Part model, mm, in its own coordinate system. A direction names the side the tool comes from. Coordinates: 2 decimals unless noted, no trailing zeros. Order: outer loops, then holes, each group sorted by start corner. A loop starts at its lowest first (then second) coordinate and runs counter-clockwise, first axis right, second up.
from build123d import *

# Parameters (mm, degrees)
SPUR_START             = -34.654843931
SPUR_GEAR_AM_OUTLINE_R = 5
SPUR_GEAR_AM_DEPTH     = 6
BOSS_EXTRUDE1_START    = -6
SKETCH2_R              = 5
SKETCH2_R_2            = 3
BOSS_EXTRUDE1_DEPTH    = 6
CUT_EXTRUDE1_REACH     = 65.242
SKETCH3_R              = 3.4


# Read off the part's stored shape, not the designer's step: spur gear_am
with BuildPart() as part:
    # spur gear_am outline → spur gear_am (new body)
    with BuildSketch(Plane.YZ.offset(SPUR_START)):
        with BuildLine():
            ThreePointArc((-3.907949552, 51.357822977), (-4.560317936, 51.46921073), (-5.215177847, 51.564867598))
            ThreePointArc((-5.215177847, 51.564867598), (-6.830693003, 49.038493172), (-7.624540457, 46.146735372))
            ThreePointArc((-7.624540457, 46.146735372), (-8.862265725, 46.181781364), (-10.099990992, 46.146735372))
            ThreePointArc((-10.099990992, 46.146735372), (-10.893838446, 49.038493172), (-12.509353602, 51.564867598))
            ThreePointArc((-12.509353602, 51.564867598), (-13.164213513, 51.46921073), (-13.816581897, 51.357822977))
            ThreePointArc((-13.816581897, 51.357822977), (-14.572335481, 48.455876478), (-14.433726972, 45.460339024))
            ThreePointArc((-14.433726972, 45.460339024), (-15.62170346, 45.111191601), (-16.788020333, 44.69538274))
            ThreePointArc((-16.788020333, 44.69538274), (-18.436616432, 47.200295486), (-20.75375528, 49.103798708))
            ThreePointArc((-20.75375528, 49.103798708), (-21.347004468, 48.810460779), (-21.933022961, 48.502931813))
            ThreePointArc((-21.933022961, 48.502931813), (-21.755036547, 45.509475985), (-20.69754004, 42.703382954))
            ThreePointArc((-20.69754004, 42.703382954), (-21.719480333, 42.004219099), (-22.700221591, 41.248349637))
            ThreePointArc((-22.700221591, 41.248349637), (-25.042190262, 43.121219015), (-27.834135107, 44.215522876))
            ThreePointArc((-27.834135107, 44.215522876), (-28.307702207, 43.753217846), (-28.770007237, 43.279650746))
            ThreePointArc((-28.770007237, 43.279650746), (-27.675703376, 40.487705901), (-25.802833998, 38.145737231))
            ThreePointArc((-25.802833998, 38.145737231), (-26.558703459, 37.164995972), (-27.257867315, 36.143055679))
            ThreePointArc((-27.257867315, 36.143055679), (-30.063960346, 37.200552186), (-33.057416174, 37.3785386))
            ThreePointArc((-33.057416174, 37.3785386), (-33.36494514, 36.792520107), (-33.658283069, 36.199270919))
            ThreePointArc((-33.658283069, 36.199270919), (-31.754779846, 33.882132071), (-29.249867101, 32.233535972))
            ThreePointArc((-29.249867101, 32.233535972), (-29.665675962, 31.067219099), (-30.014823385, 29.879242611))
            ThreePointArc((-30.014823385, 29.879242611), (-33.010360839, 30.01785112), (-35.912307338, 29.262097536))
            ThreePointArc((-35.912307338, 29.262097536), (-36.023695091, 28.609729152), (-36.119351959, 27.954869241))
            ThreePointArc((-36.119351959, 27.954869241), (-33.592977533, 26.339354085), (-30.701219732, 25.545506631))
            ThreePointArc((-30.701219732, 25.545506631), (-30.736265724, 24.307781363), (-30.701219732, 23.070056096))
            ThreePointArc((-30.701219732, 23.070056096), (-33.592977533, 22.276208642), (-36.119351959, 20.660693486))
            ThreePointArc((-36.119351959, 20.660693486), (-36.023695091, 20.005833575), (-35.912307338, 19.353465191))
            ThreePointArc((-35.912307338, 19.353465191), (-33.010360839, 18.597711607), (-30.014823385, 18.736320117))
            ThreePointArc((-30.014823385, 18.736320117), (-29.665675962, 17.548343629), (-29.249867101, 16.382026755))
            ThreePointArc((-29.249867101, 16.382026755), (-31.754779846, 14.733430656), (-33.658283069, 12.416291808))
            ThreePointArc((-33.658283069, 12.416291808), (-33.36494514, 11.82304262), (-33.057416174, 11.237024127))
            ThreePointArc((-33.057416174, 11.237024127), (-30.063960346, 11.415010541), (-27.257867315, 12.472507048))
            ThreePointArc((-27.257867315, 12.472507048), (-26.558703459, 11.450566755), (-25.802833998, 10.469825497))
            ThreePointArc((-25.802833998, 10.469825497), (-27.675703376, 8.127856826), (-28.770007237, 5.335911981))
            ThreePointArc((-28.770007237, 5.335911981), (-28.307702207, 4.862344881), (-27.834135107, 4.400039851))
            ThreePointArc((-27.834135107, 4.400039851), (-25.042190262, 5.494343712), (-22.700221591, 7.36721309))
            ThreePointArc((-22.700221591, 7.36721309), (-21.719480333, 6.611343629), (-20.69754004, 5.912179773))
            ThreePointArc((-20.69754004, 5.912179773), (-21.755036547, 3.106086742), (-21.933022961, 0.112630914))
            ThreePointArc((-21.933022961, 0.112630914), (-21.347004468, -0.194898052), (-20.75375528, -0.488235981))
            ThreePointArc((-20.75375528, -0.488235981), (-18.436616432, 1.415267242), (-16.788020333, 3.920179987))
            ThreePointArc((-16.788020333, 3.920179987), (-15.62170346, 3.504371126), (-14.433726972, 3.155223703))
            ThreePointArc((-14.433726972, 3.155223703), (-14.572335481, 0.159686249), (-13.816581897, -2.742260249))
            ThreePointArc((-13.816581897, -2.742260249), (-13.164213513, -2.853648003), (-12.509353602, -2.949304871))
            ThreePointArc((-12.509353602, -2.949304871), (-10.893838446, -0.422930445), (-10.099990992, 2.468827356))
            ThreePointArc((-10.099990992, 2.468827356), (-8.862265725, 2.433781364), (-7.624540457, 2.468827356))
            ThreePointArc((-7.624540457, 2.468827356), (-6.830693003, -0.422930445), (-5.215177847, -2.949304871))
            ThreePointArc((-5.215177847, -2.949304871), (-4.560317936, -2.853648003), (-3.907949552, -2.742260249))
            ThreePointArc((-3.907949552, -2.742260249), (-3.152195968, 0.159686249), (-3.290804477, 3.155223703))
            ThreePointArc((-3.290804477, 3.155223703), (-2.102827989, 3.504371126), (-0.936511116, 3.920179987))
            ThreePointArc((-0.936511116, 3.920179987), (0.712084983, 1.415267242), (3.029223831, -0.488235981))
            ThreePointArc((3.029223831, -0.488235981), (3.622473019, -0.194898052), (4.208491512, 0.112630914))
            ThreePointArc((4.208491512, 0.112630914), (4.030505098, 3.106086742), (2.973008591, 5.912179773))
            ThreePointArc((2.973008591, 5.912179773), (3.994948884, 6.611343629), (4.975690142, 7.36721309))
            ThreePointArc((4.975690142, 7.36721309), (7.317658813, 5.494343712), (10.109603658, 4.400039851))
            ThreePointArc((10.109603658, 4.400039851), (10.583170758, 4.862344881), (11.045475788, 5.335911981))
            ThreePointArc((11.045475788, 5.335911981), (9.951171927, 8.127856826), (8.078302549, 10.469825497))
            ThreePointArc((8.078302549, 10.469825497), (8.83417201, 11.450566755), (9.533335866, 12.472507048))
            ThreePointArc((9.533335866, 12.472507048), (12.339428897, 11.415010541), (15.332884725, 11.237024127))
            ThreePointArc((15.332884725, 11.237024127), (15.640413691, 11.82304262), (15.93375162, 12.416291808))
            ThreePointArc((15.93375162, 12.416291808), (14.030248397, 14.733430656), (11.525335652, 16.382026755))
            ThreePointArc((11.525335652, 16.382026755), (11.941144513, 17.548343629), (12.290291936, 18.736320117))
            ThreePointArc((12.290291936, 18.736320117), (15.28582939, 18.597711607), (18.187775889, 19.353465191))
            ThreePointArc((18.187775889, 19.353465191), (18.299163642, 20.005833575), (18.39482051, 20.660693486))
            ThreePointArc((18.39482051, 20.660693486), (15.868446084, 22.276208642), (12.976688283, 23.070056096))
            ThreePointArc((12.976688283, 23.070056096), (13.011734276, 24.307781363), (12.976688283, 25.545506631))
            ThreePointArc((12.976688283, 25.545506631), (15.868446084, 26.339354085), (18.39482051, 27.954869241))
            ThreePointArc((18.39482051, 27.954869241), (18.299163642, 28.609729152), (18.187775889, 29.262097536))
            ThreePointArc((18.187775889, 29.262097536), (15.28582939, 30.01785112), (12.290291936, 29.879242611))
            ThreePointArc((12.290291936, 29.879242611), (11.941144513, 31.067219099), (11.525335652, 32.233535972))
            ThreePointArc((11.525335652, 32.233535972), (14.030248397, 33.882132071), (15.93375162, 36.199270919))
            ThreePointArc((15.93375162, 36.199270919), (15.640413691, 36.792520107), (15.332884725, 37.3785386))
            ThreePointArc((15.332884725, 37.3785386), (12.339428897, 37.200552186), (9.533335866, 36.143055679))
            ThreePointArc((9.533335866, 36.143055679), (8.83417201, 37.164995972), (8.078302549, 38.145737231))
            ThreePointArc((8.078302549, 38.145737231), (9.951171927, 40.487705901), (11.045475788, 43.279650746))
            ThreePointArc((11.045475788, 43.279650746), (10.583170758, 43.753217846), (10.109603658, 44.215522876))
            ThreePointArc((10.109603658, 44.215522876), (7.317658813, 43.121219015), (4.975690142, 41.248349637))
            ThreePointArc((4.975690142, 41.248349637), (3.994948884, 42.004219099), (2.973008591, 42.703382954))
            ThreePointArc((2.973008591, 42.703382954), (4.030505098, 45.509475985), (4.208491512, 48.502931813))
            ThreePointArc((4.208491512, 48.502931813), (3.622473019, 48.810460779), (3.029223831, 49.103798708))
            ThreePointArc((3.029223831, 49.103798708), (0.712084983, 47.200295486), (-0.936511116, 44.69538274))
            ThreePointArc((-0.936511116, 44.69538274), (-2.102827989, 45.111191601), (-3.290804477, 45.460339024))
            ThreePointArc((-3.290804477, 45.460339024), (-3.152195968, 48.455876478), (-3.907949552, 51.357822977))
        make_face()
        with Locations((-8.862265724, 24.307781364)):
            Circle(SPUR_GEAR_AM_OUTLINE_R, mode=Mode.SUBTRACT)
    extrude(amount=SPUR_GEAR_AM_DEPTH)

    # Sketch2 → Boss-Extrude1 (add)
    with BuildSketch(Plane(origin=(-28.654843931, 0, 0), x_dir=(0, 0, -1), z_dir=(1, 0, 0)).offset(BOSS_EXTRUDE1_START)):
        with Locations((-24.307781364, -8.862265724)):
            Circle(SKETCH2_R)
        with Locations((-24.307781364, -8.862265724)):
            Circle(SKETCH2_R_2, mode=Mode.SUBTRACT)
    extrude(amount=BOSS_EXTRUDE1_DEPTH)

    # Sketch3 → Cut-Extrude1 (cut, up to next)
    with BuildSketch(Plane.ZY.offset(34.654843931), mode=Mode.PRIVATE) as cut_extrude1_sk1:
        with Locations((37.487332659, 0.209637475)):
            Circle(SKETCH3_R)
    cut_extrude1_tool1 = extrude(cut_extrude1_sk1.sketch, amount=-CUT_EXTRUDE1_REACH, mode=Mode.PRIVATE) & part.part
    # Sketch3 → Cut-Extrude1 (cut, up to next)
    with BuildSketch(Plane.ZY.offset(34.654843931), mode=Mode.PRIVATE) as cut_extrude1_sk2:
        with Locations((11.128230068, -17.934168924)):
            Circle(SKETCH3_R)
    cut_extrude1_tool2 = extrude(cut_extrude1_sk2.sketch, amount=-CUT_EXTRUDE1_REACH, mode=Mode.PRIVATE) & part.part
    add(cut_extrude1_tool1.solids().sort_by_distance((-34.654844, 0.209637, 37.487333))[0], mode=Mode.SUBTRACT)
    add(cut_extrude1_tool2.solids().sort_by_distance((-34.654844, -17.934169, 11.12823))[0], mode=Mode.SUBTRACT)


solid = part.part
Q1. Cut at D-D on y = -2. Write the cut outline in (x, z).
Results list:
outline: (-34.65, 3.54) - (-28.65, 3.54) - (-28.65, 34.9) - (-34.65, 34.9) - close; (-34.65, 40.07) - (-28.65, 40.07) - (-28.65, 45.08) - (-34.65, 45.08) - close
Q2. Which spindle directions (+Z, -Z, +X, -X, +Y, -Y) get a long thin tool onto all of the face, cutting with end or side? Do faces 1 (the face through (-31.697, -14.577, 0.202)), 2 (the face through (-31.7, 0.68, 1.45)), 3 (the face through (-31.697, 13.999, 33.854)), 4 (the face through (-31.7, -13.16, 51.47)), 5 (the face through (-31.697, -10.877, 49)). Say none if no direction does.
Results list:
face 1: +X, -X
face 2: -Z, +X, -X
face 3: +X, -X, +Y
face 4: +Z, +X, -X, -Y
face 5: +Z, +X, -X
Q3. Pin check, flat tips, straight feed: pin 1 Ø2 at (x, z) = (-33, 30) entering from -Y; pin 2 Ø3 at (x, z) = (-30, 10) entering from -Y. Stop position of each tip, or through.
Results list:
pin 1: stops at y = -35.96
pin 2: stops at y = -33.2
Q4. Cut at C-C on z = 1.5. Write the cut outline in (x, y).
Results list:
outline: (-34.65, -21.96) - (-28.65, -21.96) - (-28.65, -18.36) - (-34.65, -18.36) - close; (-34.65, -14.62) - (-28.65, -14.62) - (-28.65, -10.26) - (-34.65, -10.26) - close; (-34.65, -7.46) - (-28.65, -7.46) - (-28.65, -3.1) - (-34.65, -3.1) - close; (-34.65, 0.64) - (-28.65, 0.64) - (-28.65, 4.24) - (-34.65, 4.24) - close
Q5. Wall check: line 1 along Z through (x, y) = (-31.65, -26); line 2 along Y through (x, z) = (-30.25, 49); line 3 along Z through (x, y) = (-32.95, 10). Give the ranges that are in metal, low to high.
Results list:
line 1: z = 5.01 to 10.28, 10.71 to 37.9, 38.33 to 43.61
line 2: y = -20.97 to -20.58, -14.5 to -10.88, -6.85 to -3.22, 2.86 to 3.24
line 3: z = 4.43 to 8.04, 12.23 to 36.39, 40.57 to 44.19
Q6. Cut at B-B on y = -16. Write the cut outline in (x, z), and give its area (3 significant figures).
Results list:
outline: (-34.65, 3.63) - (-28.65, 3.63) - (-28.65, 8.33) - (-34.65, 8.33) - close; (-34.65, 13.92) - (-28.65, 13.92) - (-28.65, 44.98) - (-34.65, 44.98) - close
area: 215 mm2
Q7. Cut at A-A on z = 47. Write the cut outline in (x, y).
Results list:
outline: (-34.65, -21.96) - (-28.65, -21.96) - (-28.65, -18.26) - (-34.65, -18.26) - close; (-34.65, -14.62) - (-28.65, -14.62) - (-28.65, -10.24) - (-34.65, -10.24) - close; (-34.65, -7.49) - (-28.65, -7.49) - (-28.65, -3.11) - (-34.65, -3.11) - close; (-34.65, 0.54) - (-28.65, 0.54) - (-28.65, 4.23) - (-34.65, 4.23) - close
